For this review, take the finished solid that the model builds, in its own axes (mm). A direction names the side the tool comes from. Round coordinates to 2 decimals unless told otherwise and drop trailing zeros. Loops run counter-clockwise (first coordinate to the right, second up) from the corner with the lowest first, then second, coordinate; pieces in that order, holes last.
1. Consider section A-A on y = 2. State the section outline as (x, z) points, then the cut area to 3 significant figures.
2. Tool access review of faces 4 (the cylindrical face through (4.45, -4.49, 1.43)), 5 (the flat face through (27, 4, 0)): name each direction out of +Z, -Z, +X, -X, +Y, -Y from which nothing blocks a thin tool from reaching the whole face with its end or side.
3. Clearance check with a flat-ended pin moving along its axis: pin 1 Ø2.5 at (x, y) = (49, 0) entering from +Z. State where the tip first meets the part, or that it passes through.
4. Consider section B-B on x = 31. State the section outline as (y, z) points, then the cut area to 3 significant figures.
5. Consider section D-D on y = 0. State the section outline as (x, z) points, then the cut area to 3 significant figures.
6. To check wall thickness, follow line 1 along X through (y, z) = (-4.5, 0); line 2 along Y through (x, z) = (19.5, -1.5); line 3 along Y through (x, z) = (49, 4.5). State the ranges of each line that lie inside material, in increasing order.
7. Consider section C-C on x = 14. State the section outline as (y, z) points.
8. Draft analysis for pull direction Z (two halves, no side actions). For faces 1 (the flat face through (27, -5, 0)), 2 (the flat face through (27, 0, 5)), 3 (the flat face through (27, -4, 0)), state which applies: released by +Z, released by -Z, zero draft, split by the parting line, or undercut.
from build123d import *

# Parameters (mm, degrees)
SKETCH_1_W          = 10
SKETCH_1_H          = 10
SKETCH_1_W_2        = 8
SKETCH_1_H_2        = 8
EXTRUDE_1_DEPTH     = 54
SKETCH_2_R          = 1.5
CUT_EXTRUDE_1_DEPTH = 56.145262716
SKETCH_3_R          = 1.5
CUT_EXTRUDE_2_DEPTH = 56.145262716


with BuildPart() as part:
    # ｽｹｯﾁ1 → 押し出し-薄板1 (new body)
    with BuildSketch(Plane(origin=(0, 0, 0), x_dir=(0, 0, -1), z_dir=(1, 0, 0))):
        Rectangle(SKETCH_1_W, SKETCH_1_H)
        Rectangle(SKETCH_1_W_2, SKETCH_1_H_2, mode=Mode.SUBTRACT)
    extrude(amount=EXTRUDE_1_DEPTH)

    # ｽｹｯﾁ2 → ｶｯﾄ - 押し出し1 (cut, through all)
    with BuildSketch(Plane(origin=(0, 5, 0), x_dir=(1, 0, 0), z_dir=(0, 1, 0))):
        with Locations(Location((4, 0, 0), (0, 0, 270))):
            Circle(SKETCH_2_R)
        with Locations(Location((14, 0, 0), (0, 0, 270))):
            Circle(SKETCH_2_R)
        with Locations(Location((39, 0, 0), (0, 0, 270))):
            Circle(SKETCH_2_R)
    extrude(amount=-CUT_EXTRUDE_1_DEPTH, mode=Mode.SUBTRACT)

    # ｽｹｯﾁ3 → ｶｯﾄ - 押し出し2 (cut, through all)
    with BuildSketch(Plane.XY.offset(5)):
        with Locations((49, 0)):
            Circle(SKETCH_3_R)
        with Locations((29, 0)):
            Circle(SKETCH_3_R)
    extrude(amount=-CUT_EXTRUDE_2_DEPTH, mode=Mode.SUBTRACT)


solid = part.part
Resolved:
1. outline: (0, -5) - (54, -5) - (54, -4) - (0, -4) - close; (0, 4) - (54, 4) - (54, 5) - (0, 5) - close
1. area: 108 mm2
2. face 4: +Y, -Y
2. face 5: +X, -X
3. pin 1: passes through
4. outline: (-5, -5) - (5, -5) - (5, 5) - (-5, 5) - close; hole (-4, -4) - (4, -4) - (4, 4) - (-4, 4) - close
4. area: 36.0 mm2
5. outline: (0, -5) - (27.5, -5) - (27.5, -4) - (0, -4) - close; (0, 4) - (27.5, 4) - (27.5, 5) - (0, 5) - close; (30.5, -5) - (47.5, -5) - (47.5, -4) - (30.5, -4) - close; (30.5, 4) - (47.5, 4) - (47.5, 5) - (30.5, 5) - close; (50.5, -5) - (54, -5) - (54, -4) - (50.5, -4) - close; (50.5, 4) - (54, 4) - (54, 5) - (50.5, 5) - close
5. area: 96.0 mm2
6. line 1: x = 0 to 2.5, 5.5 to 12.5, 15.5 to 37.5, 40.5 to 54
6. line 2: y = -5 to -4, 4 to 5
6. line 3: y = -5 to -1.5, 1.5 to 5
7. outline: (-5, -5) - (5, -5) - (5, -1.5) - (4, -1.5) - (4, -4) - (-4, -4) - (-4, -1.5) - (-5, -1.5) - close; (-5, 1.5) - (-4, 1.5) - (-4, 4) - (4, 4) - (4, 1.5) - (5, 1.5) - (5, 5) - (-5, 5) - close
8. face 1: zero draft
8. face 2: released by +Z
8. face 3: undercut
